from build123d import *
from OCP.BRepFilletAPI import BRepFilletAPI_MakeChamfer

# Parameters (mm, degrees)
SKETCH1_W           = 0.65
SKETCH1_H           = 0.65
BOSS_EXTRUDE1_DEPTH = 11.3
CHAMFER1_SIZE       = 0.25
CHAMFER1_SIZE2      = 0.1
CHAMFER2_SIZE       = 0.1
CHAMFER2_SIZE2      = 0.25
SKETCH2_W           = 2.54
SKETCH2_H           = 2.4
BOSS_EXTRUDE2_DEPTH = 2.3
CHAMFER3_SIZE       = 0.25
SKETCH6_W           = 1.9
SKETCH6_H           = 0.2
CUT_EXTRUDE5_DEPTH  = 6
SKETCH7_W           = 0.65
SKETCH7_H           = 0.65
BOSS_EXTRUDE4_DEPTH = 3
CHAMFER5_SIZE       = 0.25
CHAMFER5_SIZE2      = 0.1


with BuildPart() as part:
    # Sketch1 → Boss-Extrude1 (new body)
    with BuildSketch(Plane(origin=(0, 0, 0), x_dir=(1, 0, 0), z_dir=(0, 1, 0))):
        with Locations((0.325, -0.325)):
            Rectangle(SKETCH1_W, SKETCH1_H)
    extrude(amount=BOSS_EXTRUDE1_DEPTH)

    # Chamfer1: one chamfer whose edges measure the first distance from different faces: ONE call of the kernel's chamfer builder (chamfer() names one face for all edges)
    chamfer1_edges_1 = [part.edges().sort_by_distance(p)[0] for p in [
        (0.65, 11.3, 0.325),
    ]]
    chamfer1_side_1 = [part.faces().sort_by_distance(p)[0] for p in [
        (0.65, 5.65, 0.325),
    ]]
    chamfer1_edges_2 = [part.edges().sort_by_distance(p)[0] for p in [
        (0.325, 11.3, 0),
    ]]
    chamfer1_side_2 = [part.faces().sort_by_distance(p)[0] for p in [
        (0.325, 5.65, 0),
    ]]
    chamfer1_edges_3 = [part.edges().sort_by_distance(p)[0] for p in [
        (0, 11.3, 0.325),
    ]]
    chamfer1_side_3 = [part.faces().sort_by_distance(p)[0] for p in [
        (0, 5.65, 0.325),
    ]]
    chamfer1_edges_4 = [part.edges().sort_by_distance(p)[0] for p in [
        (0.325, 11.3, 0.65),
    ]]
    chamfer1_side_4 = [part.faces().sort_by_distance(p)[0] for p in [
        (0.325, 5.65, 0.65),
    ]]
    chamfer1 = BRepFilletAPI_MakeChamfer(part.part.solid().wrapped)
    for e in chamfer1_edges_1:
        chamfer1.Add(CHAMFER1_SIZE, CHAMFER1_SIZE2, e.wrapped, chamfer1_side_1[0].wrapped)  # the first distance lies on this face
    for e in chamfer1_edges_2:
        chamfer1.Add(CHAMFER1_SIZE, CHAMFER1_SIZE2, e.wrapped, chamfer1_side_2[0].wrapped)  # the first distance lies on this face
    for e in chamfer1_edges_3:
        chamfer1.Add(CHAMFER1_SIZE, CHAMFER1_SIZE2, e.wrapped, chamfer1_side_3[0].wrapped)  # the first distance lies on this face
    for e in chamfer1_edges_4:
        chamfer1.Add(CHAMFER1_SIZE, CHAMFER1_SIZE2, e.wrapped, chamfer1_side_4[0].wrapped)  # the first distance lies on this face
    add(Compound.cast(chamfer1.Shape()), mode=Mode.REPLACE)

    # Chamfer2
    chamfer2_edges = [part.edges().sort_by_distance(p)[0] for p in [
        (0.325, 0, 0),
        (0.65, 0, 0.325),
        (0.325, 0, 0.65),
        (0, 0, 0.325),
    ]]
    chamfer2_side = [part.faces().sort_by_distance(p)[0] for p in [
        (0.325, 0, 0.325),
    ]]
    chamfer(chamfer2_edges, length=CHAMFER2_SIZE, length2=CHAMFER2_SIZE2, reference=chamfer2_side[0])

    # Sketch2 → Boss-Extrude2 (add)
    with BuildSketch(Plane(origin=(0, 3, 0), x_dir=(-1, 0, 0), z_dir=(0, -1, 0))):
        with Locations((-0.325, -0.325)):
            Rectangle(SKETCH2_W, SKETCH2_H)
    extrude(amount=-BOSS_EXTRUDE2_DEPTH)

    # Chamfer3
    chamfer3_edges = [part.edges().sort_by_distance(p)[0] for p in [
        (1.595, 4.15, 1.525),
        (1.595, 4.15, -0.875),
        (-0.945, 4.15, -0.875),
        (-0.945, 4.15, 1.525),
    ]]
    chamfer(chamfer3_edges, length=CHAMFER3_SIZE)

    # Sketch6 → Cut-Extrude5 (cut)
    with BuildSketch(Plane(origin=(1.595, 0, 0), x_dir=(0, 0, -1), z_dir=(1, 0, 0))):
        with Locations((-0.325, 3.1)):
            Rectangle(SKETCH6_W, SKETCH6_H)
    extrude(amount=-CUT_EXTRUDE5_DEPTH, mode=Mode.SUBTRACT)


with BuildPart() as body_2:
    # of the pieces the cut leaves, the one that is kept (cut_extrude5_keep)
    add(part.part.solids().sort_by_distance((1.345, 3, -0.875))[0])

    # Sketch7 → Boss-Extrude4 (add)
    with BuildSketch(Plane.XZ.offset(-3.2)):
        with Locations((0.325, 0.325)):
            Rectangle(SKETCH7_W, SKETCH7_H)
    extrude(amount=BOSS_EXTRUDE4_DEPTH)

    # Chamfer5: one chamfer whose edges measure the first distance from different faces: ONE call of the kernel's chamfer builder (chamfer() names one face for all edges)
    chamfer5_edges_1 = [body_2.edges().sort_by_distance(p)[0] for p in [
        (0, 0.2, 0.325),
    ]]
    chamfer5_side_1 = [body_2.faces().sort_by_distance(p)[0] for p in [
        (0, 1.7, 0.325),
    ]]
    chamfer5_edges_2 = [body_2.edges().sort_by_distance(p)[0] for p in [
        (0.325, 0.2, 0),
    ]]
    chamfer5_side_2 = [body_2.faces().sort_by_distance(p)[0] for p in [
        (0.325, 1.7, 0),
    ]]
    chamfer5_edges_3 = [body_2.edges().sort_by_distance(p)[0] for p in [
        (0.65, 0.2, 0.325),
    ]]
    chamfer5_side_3 = [body_2.faces().sort_by_distance(p)[0] for p in [
        (0.65, 1.7, 0.325),
    ]]
    chamfer5_edges_4 = [body_2.edges().sort_by_distance(p)[0] for p in [
        (0.325, 0.2, 0.65),
    ]]
    chamfer5_side_4 = [body_2.faces().sort_by_distance(p)[0] for p in [
        (0.325, 1.7, 0.65),
    ]]
    chamfer5 = BRepFilletAPI_MakeChamfer(body_2.part.solid().wrapped)
    for e in chamfer5_edges_1:
        chamfer5.Add(CHAMFER5_SIZE, CHAMFER5_SIZE2, e.wrapped, chamfer5_side_1[0].wrapped)  # the first distance lies on this face
    for e in chamfer5_edges_2:
        chamfer5.Add(CHAMFER5_SIZE, CHAMFER5_SIZE2, e.wrapped, chamfer5_side_2[0].wrapped)  # the first distance lies on this face
    for e in chamfer5_edges_3:
        chamfer5.Add(CHAMFER5_SIZE, CHAMFER5_SIZE2, e.wrapped, chamfer5_side_3[0].wrapped)  # the first distance lies on this face
    for e in chamfer5_edges_4:
        chamfer5.Add(CHAMFER5_SIZE, CHAMFER5_SIZE2, e.wrapped, chamfer5_side_4[0].wrapped)  # the first distance lies on this face
    add(Compound.cast(chamfer5.Shape()), mode=Mode.REPLACE)


solid = body_2.part
Can you work these out from the model? Positions are in its coordinate system, mm. Give positions to 0.01 mm unless a question says otherwise; leave off trailing zeros. Loops run counter-clockwise (first coordinate to the right, second up) from the corner with the lowest first, then second, coordinate; pieces in that order, holes last. Notation, with made-up numbers: (23, 8) - (44, 8) arc R21 cw to (44, 18) - close; hole circle Ø7 at (30, -31.5). An arc over 180 degrees is marked (long way). Answer as a JSON object with one key per item and string values.
Q1. If we mould it in two halves opening along Z, with no side actions, what happens to faces 1 (the flat face through (0, 5.3, 1)), 2 (the flat face through (0, 4, -0.875)), 3 (the flat face through (0, 3.2, 1))? For each: pulls with the +Z half, pulls with the -Z half, needs draft (parallel to the pull), parting line crosses it, or undercut.
Geometry says:
{"face 1": "needs draft", "face 2": "pulls with the -Z half", "face 3": "undercut"}
Q2. If I drill on L1, parallel to X at y = 7.75, z = 0.5; L2, parallel to Y at x = 1.25, z = 0.45; L3, parallel to Y at x = 0.4, z = -0.7, over which ranges is the centre line in solid material (lowest first)?
Geometry says:
{"L1": "0 to 0.65", "L2": "3.2 to 5.3", "L3": "3 to 5.3"}
Q3. Imagine slicing it at B-B on y = 4.75. Write out the boundary of the cut face in (x, z) (3 decimals).
Geometry says:
{"outline": "(-0.945, -0.625) - (-0.695, -0.875) - (1.345, -0.875) - (1.595, -0.625) - (1.595, 1.275) - (1.345, 1.525) - (-0.695, 1.525) - (-0.945, 1.275) - close"}
Q4. Imagine slicing it at A-A on x = 0.25. Write out the boundary of the cut face in (y, z) (3 decimals), plus the area to 3 significant figures.
Geometry says:
{"outline": "(0.2, 0.1) - (0.45, 0) - (3.2, 0) - (3.2, -0.625) - (3, -0.625) - (3, -0.875) - (5.3, -0.875) - (5.3, 0) - (11.05, 0) - (11.3, 0.1) - (11.3, 0.55) - (11.05, 0.65) - (5.3, 0.65) - (5.3, 1.525) - (3, 1.525) - (3, 1.275) - (3.2, 1.275) - (3.2, 0.65) - (0.45, 0.65) - (0.2, 0.55) - close", "area": "10.9 mm²"}
Q5. Will these pins go through, and if not, where does the flat tip stop? P1, Ø0.5, axis at x = 0.5, y = 9.5, coming from the +Z side; P2, Ø0.5, axis at y = 7.5, z = 0.5, coming from the -X side; P3, Ø0.7, axis at x = 0.5, y = 2, coming from the -Z side.
Geometry says:
{"P1": "z = 0.65", "P2": "x = 0", "P3": "z = 0"}
Q6. Imagine slicing it at C-C on z = 0.45. Write out the boundary of the cut face in (x, y) (3 decimals), plus the area to 3 significant figures.
Geometry says:
{"outline": "(-0.945, 3.2) - (0, 3.2) - (0, 0.45) - (0.1, 0.2) - (0.55, 0.2) - (0.65, 0.45) - (0.65, 3.2) - (1.595, 3.2) - (1.595, 5.3) - (0.65, 5.3) - (0.65, 11.05) - (0.55, 11.3) - (0.1, 11.3) - (0, 11.05) - (0, 5.3) - (-0.945, 5.3) - close", "area": "11.1 mm²"}
Q7. Imagine slicing it at D-D on x = 1.15. Write out the boundary of the cut face in (y, z) (3 decimals), plus the area to 3 significant figures.
Geometry says:
{"outline": "(3, -0.875) - (5.3, -0.875) - (5.3, 1.525) - (3, 1.525) - (3, 1.275) - (3.2, 1.275) - (3.2, -0.625) - (3, -0.625) - close", "area": "5.14 mm²"}
